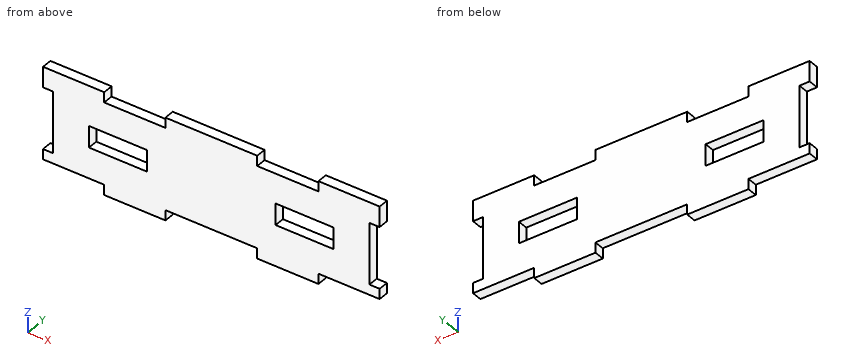
```python
from build123d import *

# Parameters (mm, degrees)
SKETCH1_W           = 28.5
SKETCH1_H           = 10.5
BOSS_EXTRUDE1_DEPTH = 5


with BuildPart() as part:
    # Sketch1 → Boss-Extrude1 (new body)
    with BuildSketch(Plane(origin=(0, 0, 0), x_dir=(1, 0, 0), z_dir=(0, 1, 0))):
        Polygon((0, 40), (0, 45), (30, 45), (30, 50), (60, 50), (60, 45), (105, 45), (105, 50), (135, 50), (135, 45), (165, 45), (165, 40), (160, 40), (160, 10), (165, 10), (165, 0), (135, 0), (135, 5), (105, 5), (105, 0), (60, 0), (60, 5), (30, 5), (30, 0), (0, 0), (0, 10), (5, 10), (5, 40), align=None)
        with Locations((36.75, 24.75)):
            Rectangle(SKETCH1_W, SKETCH1_H, mode=Mode.SUBTRACT)
        with Locations((128.25, 24.75)):
            Rectangle(SKETCH1_W, SKETCH1_H, mode=Mode.SUBTRACT)
    extrude(amount=BOSS_EXTRUDE1_DEPTH)


solid = part.part
```
Input: part model. Units: mm. Frame: model coordinates. Coordinates: 2 decimals unless noted, no trailing zeros. Write each loop counter-clockwise with the first axis right and the second up, starting at its lowest first coordinate (ties: lowest second). Pieces come first, ordered by that corner, then holes. Notation, with made-up numbers: M -24,-18.75 L 22,-18.75 A11 cw 22,-8.75 Z; hole C 26,-34 d6. An arc over 180 degrees is marked long. Use one line per item in the form item = value.
Q1. Section A-A (z = -21.5). Return loops of the section in (x, y), plus the area to 3 significant figures.
Answer below:
outline = M 5,0 L 22.5,0 L 22.5,5 L 5,5 Z; M 51,0 L 114,0 L 114,5 L 51,5 Z; M 142.5,0 L 160,0 L 160,5 L 142.5,5 Z
area = 490 mm²
Q2. First-contact query: pin 1 (1.5 mm diameter, centred on x = 15.5, y = 1.5, fed in from -Z); pin 2 (1.5 mm diameter, centred on y = 3, z = -22.5, fed in from -X); pin 3 (4 mm diameter, centred on x = 44.5, z = -27, fed in from +Y); pin 4 (2.5 mm diameter, centred on x = 39, y = 2, fed in from +Z). Flat tips, straight axial feed; report the tip coordinate or a pass-through.
Answer below:
pin_1 = -45
pin_2 = 5
pin_3 = through
pin_4 = -5
Q3. Section D-D (x = 76). Return loops of the section in (y, z).
Answer below:
outline = M 0,-45 L 5,-45 L 5,0 L 0,0 Z
Q4. Section B-B (y = 3.95). Count the separate pieces of the cut face and the enclosed holes in it, plus the area to 3 significant figures.
Answer below:
separate_pieces = 1
enclosed_holes = 2
area = 6,530 mm²
Q5. Section C-C (z = -32). Return loops of the section in (x, y).
Answer below:
outline = M 5,0 L 160,0 L 160,5 L 5,5 Z
Q6. Material intervals for probe 1 along X at (y, z) = (4.7, -26.5); probe 2 along Z at (x, y) = (32, 3); probe 3 along X at (y, z) = (3.3, -2.5), sorted ascending. Write a range as from..to.
Answer below:
probe_1 = 5..22.5, 51..114, 142.5..160
probe_2 = -50..-30, -19.5..-5
probe_3 = 0..30, 60..105, 135..165
